Verification items for this drawing (mm, ordinates from the low corner). A direction names the side the tool comes from. Round coordinates to 2 decimals unless told otherwise and drop trailing zeros. Order: outer loops, then holes, each group sorted by start corner. A loop starts at its lowest first (then second) coordinate and runs counter-clockwise, first axis right, second up.
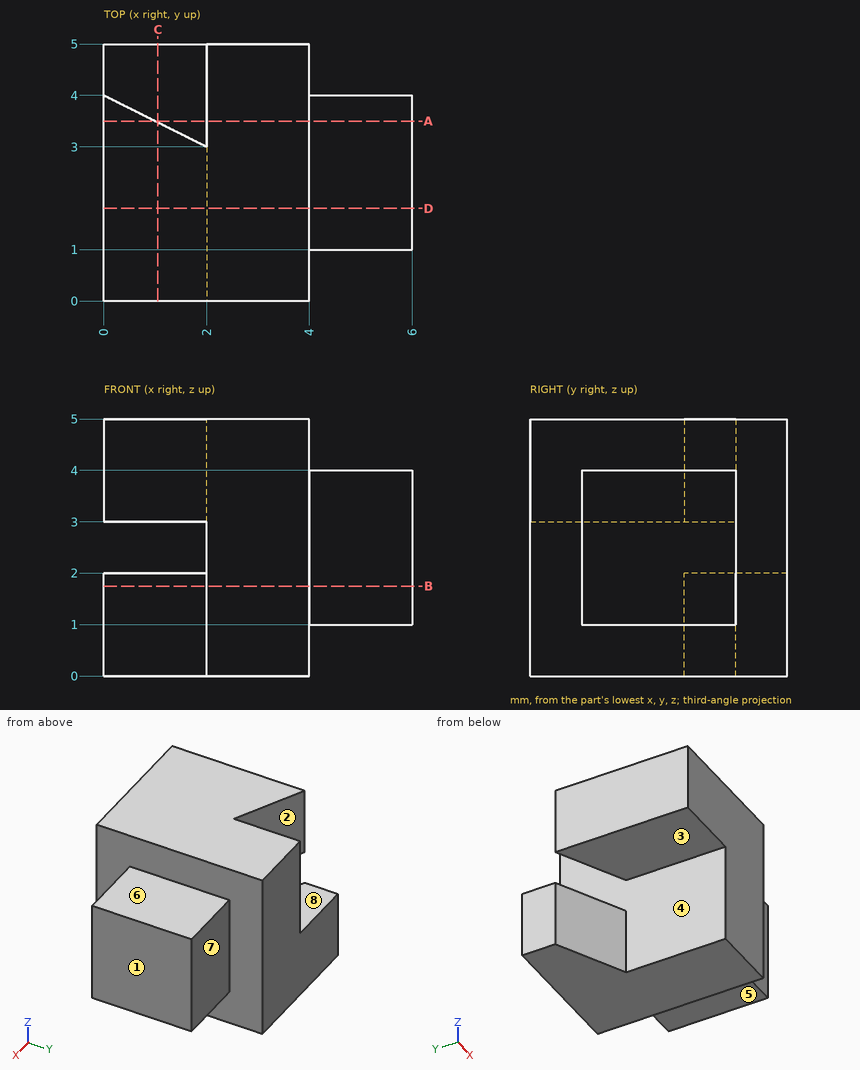
Item 1: Sectioned sample at B-B (z = 1.75). Record the cut outline in (x, y).
Answer:
outline: (0, 4) - (2, 3) - (2, 0) - (4, 0) - (4, 1) - (6, 1) - (6, 4) - (4, 4) - (4, 5) - (0, 5) - close
Item 2: Go/stop test with flat-tipped pins: P1, Ø0.6, axis at x = 5, z = 3, coming from the -Y side; P2, Ø1, axis at x = 5.5, y = 2, coming from the -Z side; P3, Ø2, axis at y = 1, z = 1.5, coming from the -X side. Record where each tip stops, or that it passes through.
Answer:
P1: stops at y = 1
P2: stops at z = 1
P3: stops at x = 2
Item 3: Sectioned sample at C-C (x = 1.05). Record the cut outline in (y, z) (3 decimals).
Answer:
outline: (0, 3) - (3.475, 3) - (3.475, 5) - (0, 5) - close; (3.475, 0) - (5, 0) - (5, 2) - (3.475, 2) - close
Item 4: Release check for a two-part mould opening along X. For the marked faces 1, 2 and 3 record: released by +X, released by -X, zero draft, split by the parting line, or undercut.
Answer:
face 1: released by +X
face 2: undercut
face 3: zero draft
Item 5: Access from +Z, -Z, +X, -X, +Y, -Y to the whole of each face (thin tool, end or side, straight path). Record for the marked faces 4, 5, 6, 7 and 8.
Answer:
face 4: none
face 5: -Z, +X, +Y, -Y
face 6: +Z, +X, +Y, -Y
face 7: +Z, -Z, +X, +Y
face 8: +Z, -X, +Y, -Y
Item 6: Sectioned sample at A-A (y = 3.5). Record the cut outline in (x, z), and give its area (3 significant figures).
Answer:
outline: (0, 3) - (1, 3) - (1, 5) - (0, 5) - close; (1, 0) - (4, 0) - (4, 1) - (6, 1) - (6, 4) - (4, 4) - (4, 5) - (2, 5) - (2, 2) - (1, 2) - close
area: 20.0 mm2
Item 7: Scan lines: line 1 along X through (y, z) = (1.75, 1.15); line 2 along X through (y, z) = (3.25, 3.45); line 3 along X through (y, z) = (3.4, 3.2). Record each from-to range of solid material in increasing order.
Answer:
line 1: x = 2 to 6
line 2: x = 0 to 1.5, 2 to 6
line 3: x = 0 to 1.2, 2 to 6
Item 8: Sectioned sample at D-D (y = 1.8). Record the cut outline in (x, z).
Answer:
outline: (0, 3) - (2, 3) - (2, 0) - (4, 0) - (4, 1) - (6, 1) - (6, 4) - (4, 4) - (4, 5) - (0, 5) - close
